Part model, mm, in its own coordinate system. A direction names the side the tool comes from. Coordinates: 2 decimals unless noted, no trailing zeros. Loops run counter-clockwise (first coordinate to the right, second up) from the corner with the lowest first, then second, coordinate; pieces in that order, holes last. Notation, with made-up numbers: (64.5, -24.75) - (71.5, -24.75) arc R22 cw to (71.5, 10.25) - close; hole circle Ø8 at (48, 41.25). An arc over 180 degrees is marked (long way). Use a Markdown table: item, result. Add a question column.
1. Pull direction Y, two halves, no side cores. Call faces 1 (the cylindrical face through (11.475, -12.2, 3.131)), 2 (the flat face through (-19, 4.749, 3)), 3 (the flat face through (19, -4.749, 3)): pulls with the +Y half, pulls with the -Y half, needs draft (parallel to the pull), parting line crosses it, or undercut.
2. Band-saw the part on B-B, the plane z = 1.25. Count the separate pieces of the cut face and the enclosed holes in it, plus the area to 3 significant figures.
3. Wall check: probe 1 along X at (y, z) = (-0.5, 4.25); probe 2 along Y at (x, z) = (-8.5, 1.5); probe 3 along X at (y, z) = (1, 5). Give the ranges that are in metal, low to high. Write a range as [from, to].
4. Band-saw the part on C-C, the plane x = 21. Give the cut face in (y, z), plus the area to 3 significant figures.
5. Band-saw the part on A-A, the plane x = 34. Give the cut face in (y, z).
6. Drop flat-ended pins along their axis: pin 1 (1.2 mm diameter, centred on y = 4, z = 2.5, fed in from -X); pin 2 (3 mm diameter, centred on y = 6.5, z = 4, fed in from -X); pin 3 (1.2 mm diameter, centred on x = -4, z = 4.5, fed in from -Y). Give the stop position or say it passes through.
7. 3-axis set-ups, long thin cutter, end or side, ignore diameter. For faces 4 (the flat face through (-3.994, 19, 3)), 5 (the flat face through (-19, -3.994, 3)), 6 (the flat face through (3.994, -19, 3)), 7 (the cylindrical face through (-12.2, -11.475, 3.131)): which of +Z, -Z, +X, -X, +Y, -Y reach the whole face in a straight line?
8. Band-saw the part on D-D, the plane y = -34.5. Give the cut face in (x, z).
from build123d import *

# Parameters (mm, degrees)
F1_DEPTH = 6.35
F2_W     = 7.482951507
F2_H     = 8.058561245
F3_DEPTH = 59.436
F2_R     = 6.0344313248
F4_DEPTH = 108.458


with BuildPart() as f1:
    # F0 (on Top) → F1 (new body)
    with BuildSketch(Plane.XY):
        with BuildLine():
            ThreePointArc((16.061134272, -4.7487956472), (16.5757420089, -2.3991396488), (16.7484654282, 0))
            ThreePointArc((16.7484654282, 0), (16.627209939, 2.0117116707), (16.2651992014, 3.9942945733))
            Line((16.2651992014, 3.9942945733), (16.061134272, -4.7487956472))
        make_face()
        with BuildLine():
            ThreePointArc((16.2651992014, 3.9942945733), (16.627209939, 2.0117116707), (16.7484654282, 0))
            ThreePointArc((16.7484654282, 0), (16.5757420089, -2.3991396488), (16.061134272, -4.7487956472))
            Line((16.061134272, -4.7487956472), (22.0171436027, -4.7487956472))
            Line((22.0171436027, -4.7487956472), (22.0171436027, -3.2589072692))
            ThreePointArc((22.0171436027, -3.2589072692), (21.4715103831, 0), (22.0171436027, 3.2589072692))
            Line((22.0171436027, 3.2589072692), (22.0171436027, 3.9942945733))
            Line((22.0171436027, 3.9942945733), (16.2651992014, 3.9942945733))
        make_face()
        with BuildLine():
            Line((16.061134272, -4.7487956472), (16.2651992014, 3.9942945733))
            ThreePointArc((16.2651992014, 3.9942945733), (12.1160699054, 11.5633880956), (4.7487956472, 16.061134272))
            Line((4.7487956472, 16.061134272), (-3.9942945733, 16.2651992014))
            ThreePointArc((-3.9942945733, 16.2651992014), (-11.5633880956, 12.1160699054), (-16.061134272, 4.7487956472))
            Line((-16.061134272, 4.7487956472), (-16.2651992014, -3.9942945733))
            ThreePointArc((-16.2651992014, -3.9942945733), (-12.1160699054, -11.5633880956), (-4.7487956472, -16.061134272))
            Line((-4.7487956472, -16.061134272), (3.9942945733, -16.2651992014))
            ThreePointArc((3.9942945733, -16.2651992014), (11.5633880956, -12.1160699054), (16.061134272, -4.7487956472))
        make_face()
        with BuildLine():
            Line((-3.9942945733, 16.2651992014), (4.7487956472, 16.061134272))
            ThreePointArc((4.7487956472, 16.061134272), (0.3908050556, 16.7439053273), (-3.9942945733, 16.2651992014))
        make_face()
        with BuildLine():
            ThreePointArc((-3.9942945733, 16.2651992014), (0.3908050556, 16.7439053273), (4.7487956472, 16.061134272))
            Line((4.7487956472, 16.061134272), (4.7487956472, 22.0171436027))
            Line((4.7487956472, 22.0171436027), (3.2589072692, 22.0171436027))
            ThreePointArc((3.2589072692, 22.0171436027), (0, 21.4715103831), (-3.2589072692, 22.0171436027))
            Line((-3.2589072692, 22.0171436027), (-3.9942945733, 22.0171436027))
            Line((-3.9942945733, 22.0171436027), (-3.9942945733, 16.2651992014))
        make_face()
        with BuildLine():
            Line((3.9942945733, -22.0171436027), (3.9942945733, -16.2651992014))
            ThreePointArc((3.9942945733, -16.2651992014), (-0.3908050556, -16.7439053273), (-4.7487956472, -16.061134272))
            Line((-4.7487956472, -16.061134272), (-4.7487956472, -22.0171436027))
            Line((-4.7487956472, -22.0171436027), (-3.2589072692, -22.0171436027))
            ThreePointArc((-3.2589072692, -22.0171436027), (0, -21.4715103831), (3.2589072692, -22.0171436027))
            Line((3.2589072692, -22.0171436027), (3.9942945733, -22.0171436027))
        make_face()
        with BuildLine():
            ThreePointArc((-4.7487956472, -16.061134272), (-0.3908050556, -16.7439053273), (3.9942945733, -16.2651992014))
            Line((3.9942945733, -16.2651992014), (-4.7487956472, -16.061134272))
        make_face()
        with BuildLine():
            ThreePointArc((41.4816413794, 0), (33.1287102734, 9.8677144047), (22.0171436027, 3.2589072692))
            Line((22.0171436027, 3.2589072692), (22.0171436027, -3.2589072692))
            ThreePointArc((22.0171436027, -3.2589072692), (33.1287102734, -9.8677144047), (41.4816413794, 0))
        make_face()
        with BuildLine():
            Line((22.0171436027, -3.2589072692), (22.0171436027, 3.2589072692))
            ThreePointArc((22.0171436027, 3.2589072692), (21.4715103831, 0), (22.0171436027, -3.2589072692))
        make_face()
        with BuildLine():
            Line((-16.2651992014, -3.9942945733), (-16.061134272, 4.7487956472))
            ThreePointArc((-16.061134272, 4.7487956472), (-16.7439053273, 0.3908050556), (-16.2651992014, -3.9942945733))
        make_face()
        with BuildLine():
            ThreePointArc((-16.2651992014, -3.9942945733), (-16.7439053273, 0.3908050556), (-16.061134272, 4.7487956472))
            Line((-16.061134272, 4.7487956472), (-22.0171436027, 4.7487956472))
            Line((-22.0171436027, 4.7487956472), (-22.0171436027, 3.2589072692))
            ThreePointArc((-22.0171436027, 3.2589072692), (-21.6088614766, 1.6521343922), (-21.4715103831, 0))
            ThreePointArc((-21.4715103831, 0), (-21.6088614766, -1.6521343922), (-22.0171436027, -3.2589072692))
            Line((-22.0171436027, -3.2589072692), (-22.0171436027, -3.9942945733))
            Line((-22.0171436027, -3.9942945733), (-16.2651992014, -3.9942945733))
        make_face()
        with BuildLine():
            ThreePointArc((-3.2589072692, 22.0171436027), (0, 21.4715103831), (3.2589072692, 22.0171436027))
            Line((3.2589072692, 22.0171436027), (-3.2589072692, 22.0171436027))
        make_face()
        with BuildLine():
            Line((-3.2589072692, 22.0171436027), (3.2589072692, 22.0171436027))
            ThreePointArc((3.2589072692, 22.0171436027), (8.1457632025, 25.667283543), (10.0050654981, 31.4765758812))
            ThreePointArc((10.0050654981, 31.4765758812), (-5.8092923382, 39.6223390837), (-3.2589072692, 22.0171436027))
        make_face()
        with BuildLine():
            ThreePointArc((10.0050654981, -31.4765758812), (8.1457632025, -25.667283543), (3.2589072692, -22.0171436027))
            Line((3.2589072692, -22.0171436027), (-3.2589072692, -22.0171436027))
            ThreePointArc((-3.2589072692, -22.0171436027), (-5.8092923382, -39.6223390837), (10.0050654981, -31.4765758812))
        make_face()
        with BuildLine():
            Line((-3.2589072692, -22.0171436027), (3.2589072692, -22.0171436027))
            ThreePointArc((3.2589072692, -22.0171436027), (0, -21.4715103831), (-3.2589072692, -22.0171436027))
        make_face()
        with BuildLine():
            ThreePointArc((-21.4715103831, 0), (-21.6088614766, 1.6521343922), (-22.0171436027, 3.2589072692))
            Line((-22.0171436027, 3.2589072692), (-22.0171436027, -3.2589072692))
            ThreePointArc((-22.0171436027, -3.2589072692), (-21.6088614766, -1.6521343922), (-21.4715103831, 0))
        make_face()
        with BuildLine():
            Line((-22.0171436027, -3.2589072692), (-22.0171436027, 3.2589072692))
            ThreePointArc((-22.0171436027, 3.2589072692), (-41.4816413794, 0), (-22.0171436027, -3.2589072692))
        make_face()
    extrude(amount=F1_DEPTH)

    # F2 (on face) → F3 (cut)
    with BuildSketch(Plane.XY.offset(6.35)):
        with Locations((-31.5147312358, -0.1439027255)):
            Rectangle(F2_W, F2_H)
    extrude(amount=-F3_DEPTH, mode=Mode.SUBTRACT)

    # F2 (on face) → F4 (cut)
    with BuildSketch(Plane.XY.offset(6.35)):
        with Locations((31.4765758812, 0)):
            Circle(F2_R)
        Polygon((3.2589072692, 29.9774594605), (0, 38.620531559), (-4.6109691992, 29.9774594605), align=None)
    extrude(amount=-F4_DEPTH, mode=Mode.SUBTRACT)


solid = f1.part
Geometry check:
| question | item | result |
|---|---|---|
| 1 | face 1 | undercut |
| 1 | face 2 | pulls with the +Y half |
| 1 | face 3 | pulls with the -Y half |
| 2 | separate pieces | 1 |
| 2 | enclosed holes | 3 |
| 2 | area | 2,110 mm^2 |
| 3 | probe 1 | x = [-41.47, -35.26], [-27.77, 25.46], [37.49, 41.47] |
| 3 | probe 2 | y = [-36.75, -26.2], [-14.43, 14.43], [26.2, 36.75] |
| 3 | probe 3 | x = [-41.43, -35.26], [-27.77, 25.53], [37.43, 41.43] |
| 4 | outline | (-4.75, 0) - (3.99, 0) - (3.99, 6.35) - (-4.75, 6.35) - close |
| 4 | area | 55.5 mm^2 |
| 5 | outline | (-9.68, 0) - (-5.48, 0) - (-5.48, 6.35) - (-9.68, 6.35) - close; (5.48, 0) - (9.68, 0) - (9.68, 6.35) - (5.48, 6.35) - close |
| 6 | pin 1 | stops at x = -40.89 |
| 6 | pin 2 | stops at x = -40.14 |
| 6 | pin 3 | stops at y = -40.89 |
| 7 | face 4 | +Z, -Z, -X |
| 7 | face 5 | +Z, -Z, -Y |
| 7 | face 6 | +Z, -Z, +X |
| 7 | face 7 | +Z, -Z |
| 8 | outline | (-9.54, 0) - (9.54, 0) - (9.54, 6.35) - (-9.54, 6.35) - close |
